from build123d import *

# Parameters (mm, degrees)
SKETCH_1_R          = 140
EXTRUDE_1_DEPTH     = 100
SKETCH_2_R          = 105
CUT_EXTRUDE_1_DEPTH = 100
SKETCH_3_R          = 20
EXTRUDE_2_DEPTH     = 100
SKETCH_4_R          = 130
CUT_EXTRUDE_2_DEPTH = 10
CUT_EXTRUDE_START   = -10
SKETCH_5_R          = 130
CUT_EXTRUDE_3_DEPTH = 10
CUT_EXTRUDE_4_DEPTH = 218.485631709
SKETCH_7_W          = 8
SKETCH_7_H          = 10
SKETCH_7_W_2        = 10
SKETCH_7_H_2        = 8
EXTRUDE_3_DEPTH     = 70
EXTRUDE_4_DEPTH     = 70
FILLET_3_R          = 5
CHAMFER_1_SIZE      = 10
CUT_EXTRUDE_6_DEPTH = 235.447678383
FILLET_4_R          = 10


with BuildPart() as part:
    # 草图1 → 凸台-拉伸1 (new body)
    with BuildSketch(Plane.XY):
        Circle(SKETCH_1_R)
    extrude(amount=EXTRUDE_1_DEPTH)

    # 草图2 → 切除-拉伸1 (cut)
    with BuildSketch(Plane.XY.offset(100)):
        Circle(SKETCH_2_R)
    extrude(amount=-CUT_EXTRUDE_1_DEPTH, mode=Mode.SUBTRACT)

    # 草图3 → 凸台-拉伸2 (add, through all)
    with BuildSketch(Plane.XY.offset(100)):
        with Locations((0, 115)):
            Circle(SKETCH_3_R)
        with Locations((57.5, 99.592921435)):
            Circle(SKETCH_3_R)
        with Locations((99.592921435, 57.5)):
            Circle(SKETCH_3_R)
        with Locations((115, 0)):
            Circle(SKETCH_3_R)
        with Locations((99.592921435, -57.5)):
            Circle(SKETCH_3_R)
        with Locations((57.5, -99.592921435)):
            Circle(SKETCH_3_R)
        with Locations((0, -115)):
            Circle(SKETCH_3_R)
        with Locations((-57.5, -99.592921435)):
            Circle(SKETCH_3_R)
        with Locations((-99.592921435, -57.5)):
            Circle(SKETCH_3_R)
        with Locations((-115, 0)):
            Circle(SKETCH_3_R)
        with Locations((-99.592921435, 57.5)):
            Circle(SKETCH_3_R)
        with Locations((-57.5, 99.592921435)):
            Circle(SKETCH_3_R)
    extrude(amount=-EXTRUDE_2_DEPTH)

    # 草图4 → 切除-拉伸2 (cut)
    with BuildSketch(Plane.XY.offset(100)):
        Circle(SKETCH_4_R)
    extrude(amount=-CUT_EXTRUDE_2_DEPTH, mode=Mode.SUBTRACT)

    # 草图5 → 切除-拉伸3 (cut)
    with BuildSketch(Plane(origin=(0, 0, 0), x_dir=(-1, 0, 0), z_dir=(0, 0, -1)).offset(CUT_EXTRUDE_START)):
        with Locations(Location((0, 0, 0), (0, 0, 180))):
            Circle(SKETCH_5_R)
    extrude(amount=CUT_EXTRUDE_3_DEPTH, mode=Mode.SUBTRACT)

    # 草图6 → 切除-拉伸4 (cut, through all)
    with BuildSketch(Plane.XY.offset(90)):
        Polygon((55.132863896, 95.492921435), (59.867136104, 95.492921435), (62.234272207, 99.592921435), (59.867136104, 103.692921435), (55.132863896, 103.692921435), (52.765727793, 99.592921435), align=None)
        Polygon((0, 110.265727793), (4.1, 112.632863896), (4.1, 117.367136104), (0, 119.734272207), (-4.1, 117.367136104), (-4.1, 112.632863896), align=None)
        Polygon((95.492921435, 55.132863896), (99.592921435, 52.765727793), (103.692921435, 55.132863896), (103.692921435, 59.867136104), (99.592921435, 62.234272207), (95.492921435, 59.867136104), align=None)
        Polygon((110.265727793, 0), (112.632863896, -4.1), (117.367136104, -4.1), (119.734272207, 0), (117.367136104, 4.1), (112.632863896, 4.1), align=None)
        Polygon((95.492921435, -55.132863896), (95.492921435, -59.867136104), (99.592921435, -62.234272207), (103.692921435, -59.867136104), (103.692921435, -55.132863896), (99.592921435, -52.765727793), align=None)
        Polygon((55.132863896, -95.492921435), (52.765727793, -99.592921435), (55.132863896, -103.692921435), (59.867136104, -103.692921435), (62.234272207, -99.592921435), (59.867136104, -95.492921435), align=None)
        Polygon((0, -110.265727793), (-4.1, -112.632863896), (-4.1, -117.367136104), (0, -119.734272207), (4.1, -117.367136104), (4.1, -112.632863896), align=None)
        Polygon((-55.132863896, -95.492921435), (-59.867136104, -95.492921435), (-62.234272207, -99.592921435), (-59.867136104, -103.692921435), (-55.132863896, -103.692921435), (-52.765727793, -99.592921435), align=None)
        Polygon((-95.492921435, -55.132863896), (-99.592921435, -52.765727793), (-103.692921435, -55.132863896), (-103.692921435, -59.867136104), (-99.592921435, -62.234272207), (-95.492921435, -59.867136104), align=None)
        Polygon((-110.265727793, 0), (-112.632863896, 4.1), (-117.367136104, 4.1), (-119.734272207, 0), (-117.367136104, -4.1), (-112.632863896, -4.1), align=None)
        Polygon((-95.492921435, 55.132863896), (-95.492921435, 59.867136104), (-99.592921435, 62.234272207), (-103.692921435, 59.867136104), (-103.692921435, 55.132863896), (-99.592921435, 52.765727793), align=None)
        Polygon((-55.132863896, 95.492921435), (-52.765727793, 99.592921435), (-55.132863896, 103.692921435), (-59.867136104, 103.692921435), (-62.234272207, 99.592921435), (-59.867136104, 95.492921435), align=None)
    extrude(amount=-CUT_EXTRUDE_4_DEPTH, mode=Mode.SUBTRACT)

    # 草图7 → 凸台-拉伸3 (add)
    with BuildSketch(Plane.XY.offset(100)):
        Polygon((66.507321123, 123.19405926), (73.435524353, 119.19405926), (78.435524353, 127.854313298), (71.507321123, 131.854313298), align=None)
        with Locations((0, 144.942845476)):
            Rectangle(SKETCH_7_W, SKETCH_7_H)
        Polygon((119.19405926, 73.435524353), (123.19405926, 66.507321123), (131.854313298, 71.507321123), (127.854313298, 78.435524353), align=None)
        with Locations((144.942845476, 0)):
            Rectangle(SKETCH_7_W_2, SKETCH_7_H_2)
        Polygon((123.19405926, -66.507321123), (119.19405926, -73.435524353), (127.854313298, -78.435524353), (131.854313298, -71.507321123), align=None)
        Polygon((73.435524353, -119.19405926), (66.507321123, -123.19405926), (71.507321123, -131.854313298), (78.435524353, -127.854313298), align=None)
        with Locations((0, -144.942845476)):
            Rectangle(SKETCH_7_W, SKETCH_7_H)
        Polygon((-66.507321123, -123.19405926), (-73.435524353, -119.19405926), (-78.435524353, -127.854313298), (-71.507321123, -131.854313298), align=None)
        Polygon((-119.19405926, -73.435524353), (-123.19405926, -66.507321123), (-131.854313298, -71.507321123), (-127.854313298, -78.435524353), align=None)
        with Locations((-144.942845476, 0)):
            Rectangle(SKETCH_7_W_2, SKETCH_7_H_2)
        Polygon((-123.19405926, 66.507321123), (-119.19405926, 73.435524353), (-127.854313298, 78.435524353), (-131.854313298, 71.507321123), align=None)
        Polygon((-73.435524353, 119.19405926), (-66.507321123, 123.19405926), (-71.507321123, 131.854313298), (-78.435524353, 127.854313298), align=None)
    extrude(amount=-EXTRUDE_3_DEPTH)

    # 草图9 → 凸台-拉伸4 (add)
    with BuildSketch(Plane(origin=(0, 0, 0), x_dir=(-1, 0, 0), z_dir=(0, 0, -1))):
        Polygon((34.944360781, 145.868943093), (32.35617033, 136.20968483), (40.08357694, 134.13913247), (42.671767391, 143.798390732), align=None)
        Polygon((101.78296214, 96.12610789), (108.854029951, 103.197175702), (103.197175702, 108.854029951), (96.12610789, 101.78296214), align=None)
        Polygon((136.20968483, 32.35617033), (145.868943093, 34.944360781), (143.798390732, 42.671767391), (134.13913247, 40.08357694), align=None)
        Polygon((134.13913247, -40.08357694), (143.798390732, -42.671767391), (145.868943093, -34.944360781), (136.20968483, -32.35617033), align=None)
        Polygon((96.12610789, -101.78296214), (103.197175702, -108.854029951), (108.854029951, -103.197175702), (101.78296214, -96.12610789), align=None)
        Polygon((32.35617033, -136.20968483), (34.944360781, -145.868943093), (42.671767391, -143.798390732), (40.08357694, -134.13913247), align=None)
        Polygon((-40.08357694, -134.13913247), (-42.671767391, -143.798390732), (-34.944360781, -145.868943093), (-32.35617033, -136.20968483), align=None)
        Polygon((-101.78296214, -96.12610789), (-108.854029951, -103.197175702), (-103.197175702, -108.854029951), (-96.12610789, -101.78296214), align=None)
        Polygon((-136.20968483, -32.35617033), (-145.868943093, -34.944360781), (-143.798390732, -42.671767391), (-134.13913247, -40.08357694), align=None)
        Polygon((-134.13913247, 40.08357694), (-143.798390732, 42.671767391), (-145.868943093, 34.944360781), (-136.20968483, 32.35617033), align=None)
        Polygon((-96.12610789, 101.78296214), (-103.197175702, 108.854029951), (-108.854029951, 103.197175702), (-101.78296214, 96.12610789), align=None)
        Polygon((-32.35617033, 136.20968483), (-34.944360781, 145.868943093), (-42.671767391, 143.798390732), (-40.08357694, 134.13913247), align=None)
    extrude(amount=-EXTRUDE_4_DEPTH)

    # 圆角3
    fillet_3_edges = [part.edges().sort_by_distance(p)[0] for p in [
        (70, 121.24355653, 30),
        (-70, 121.24355653, 30),
        (-121.24355653, 70, 30),
        (-140, 0, 30),
        (0, 140, 30),
        (121.24355653, 70, 30),
        (139.98571064, 2.000204155, 30),
        (121.24355653, -70, 30),
        (70, -121.24355653, 30),
        (0, -140, 30),
        (-70, -121.24355653, 30),
        (-121.24355653, -70, 30),
        (-119.19405926, -73.435524353, 65),
        (-123.19405926, -66.507321123, 65),
        (-66.507321123, -123.19405926, 65),
        (-73.435524353, -119.19405926, 65),
        (4, -139.942845476, 65),
        (-4, -139.942845476, 65),
        (73.435524353, -119.19405926, 65),
        (66.507321123, -123.19405926, 65),
        (123.19405926, -66.507321123, 65),
        (119.19405926, -73.435524353, 65),
        (139.942845476, 4, 65),
        (139.942845476, -4, 65),
        (119.19405926, 73.435524353, 65),
        (123.19405926, 66.507321123, 65),
        (-4, 139.942845476, 65),
        (4, 139.942845476, 65),
        (-139.942845476, -4, 65),
        (-139.942845476, 4, 65),
        (-123.19405926, 66.507321123, 65),
        (-119.19405926, 73.435524353, 65),
        (-73.435524353, 119.19405926, 65),
        (-66.507321123, 123.19405926, 65),
        (66.507321123, 123.19405926, 65),
        (73.435524353, 119.19405926, 65),
        (-36.234666314, 135.22961568, 70),
        (36.234666314, 135.22961568, 70),
        (98.994949366, 98.994949366, 70),
        (135.22961568, 36.234666314, 70),
        (135.22961568, -36.234666314, 70),
        (98.994949366, -98.994949366, 70),
        (36.234666314, -135.22961568, 70),
        (-36.234666314, -135.22961568, 70),
        (-98.994949366, -98.994949366, 70),
        (-135.22961568, -36.234666314, 70),
        (-135.22961568, 36.234666314, 70),
        (-98.994949366, 98.994949366, 70),
        (-96.12610789, 101.78296214, 35),
        (-101.78296214, 96.12610789, 35),
        (-134.13913247, 40.08357694, 35),
        (-136.20968483, 32.35617033, 35),
        (-136.20968483, -32.35617033, 35),
        (-134.13913247, -40.08357694, 35),
        (-101.78296214, -96.12610789, 35),
        (-96.12610789, -101.78296214, 35),
        (-40.08357694, -134.13913247, 35),
        (-32.35617033, -136.20968483, 35),
        (32.35617033, -136.20968483, 35),
        (40.08357694, -134.13913247, 35),
        (96.12610789, -101.78296214, 35),
        (101.78296214, -96.12610789, 35),
        (134.13913247, -40.08357694, 35),
        (136.20968483, -32.35617033, 35),
        (136.20968483, 32.35617033, 35),
        (134.13913247, 40.08357694, 35),
        (101.78296214, 96.12610789, 35),
        (96.12610789, 101.78296214, 35),
        (40.08357694, 134.13913247, 35),
        (32.35617033, 136.20968483, 35),
        (-40.08357694, 134.13913247, 35),
        (-32.35617033, 136.20968483, 35),
    ]]
    fillet(fillet_3_edges, radius=FILLET_3_R)

    # 倒角1
    chamfer_1_edges = [part.edges().sort_by_distance(p)[0] for p in [
        (74.971422738, 129.854313298, 100),
        (106.025602827, 106.025602827, 0),
        (129.854313298, 74.971422738, 100),
        (144.833666913, 38.808064086, 0),
        (149.942845476, 0, 100),
        (144.833666913, -38.808064086, 0),
        (129.854313298, -74.971422738, 100),
        (106.025602827, -106.025602827, 0),
        (74.971422738, -129.854313298, 100),
        (38.808064086, -144.833666913, 0),
        (0, -149.942845476, 100),
        (-38.808064086, -144.833666913, 0),
        (-74.971422738, -129.854313298, 100),
        (-106.025602827, -106.025602827, 0),
        (-129.854313298, -74.971422738, 100),
        (-144.833666913, -38.808064086, 0),
        (-149.942845476, 0, 100),
        (-129.854313298, 74.971422738, 100),
        (-74.971422738, 129.854313298, 100),
        (0, 149.942845476, 100),
        (-144.833666913, 38.808064086, 0),
        (-106.025602827, 106.025602827, 0),
        (-38.808064086, 144.833666913, 0),
        (38.808064086, 144.833666913, 0),
    ]]
    chamfer(chamfer_1_edges, length=CHAMFER_1_SIZE)

    # 草图10 → 切除-拉伸6 (cut, through all)
    with BuildSketch(Plane(origin=(0, 0, 0), x_dir=(-1, 0, 0), z_dir=(0, 0, -1))):
        with BuildLine():
            Line((0, 0), (25.926748518, 162.950310559))
            ThreePointArc((25.926748518, 162.950310559), (59.021932425, -154.082482758), (-128.15573424, 103.928378134))
            Line((-128.15573424, 103.928378134), (0, 0))
        make_face()
    extrude(amount=-CUT_EXTRUDE_6_DEPTH, mode=Mode.SUBTRACT)

    # 圆角4
    fillet_4_edges = [part.edges().sort_by_distance(p)[0] for p in [
        (81.553649062, 66.136240631, 50),
        (-16.498839966, 103.695652174, 50),
    ]]
    fillet(fillet_4_edges, radius=FILLET_4_R)


solid = part.part
Can you work these out from the model? Positions are in its coordinate system, mm. A direction names the side the tool comes from. Coordinates: 2 decimals unless noted, no trailing zeros. Loops run counter-clockwise (first coordinate to the right, second up) from the corner with the lowest first, then second, coordinate; pieces in that order, holes last. Notation, with made-up numbers: (16, 40.5) - (37, 40.5) arc R25 cw to (37, 55.5) - close; hole circle Ø9 at (55.25, 49.5). An arc over 180 degrees is marked (long way). Answer as a JSON object with one key per item and string values. Group by question number.
Item 1: If we section it at B-B (x = 10.5): List the corners of the cut face in (y, z) for me, plus the area to 3 significant figures.
Item 2: On a 3-axis mill with a long thin cutter (end or side, diameter ignored), from which of +Z, -Z, +X, -X, +Y, -Y can I reach the whole of each face in a straight line? I mean faces 1 (the face through (-4, 147, 63)), 2 (the face through (104, 104, 70)), 3 (the face through (71.01, 77.347, 50.56)), 4 (the face through (-4.1, 115, 51)). Say none if no direction works.
Item 3: If we section it at A-A (z = 11.5): State how many separate pieces and enclosed holes the cut face has, plus the area to 3 significant figures.
Item 4: For pin 1 (2 mm diameter, centred on x = 39.5, y = 143, fed in from +Z); pin 2 (12 mm diameter, centred on y = 117.5, z = 12.5, fed in from +X); pin 3 (4 mm diameter, centred on x = 57.5, z = 44, fed in from -Y); pin 4 (1.5 mm diameter, centred on x = -1.5, y = 140.5, fed in from +Z), each with a flat end and sliding along its axis, tell me the tip position at first contact or that it passes through.
Item 5: If we mould it in two halves opening along Y, with no side actions, what happens to faces 5 (the face through (65.96, 125.03, 61.98)), 6 (the face through (61.07, 101.61, 50.56)), 7 (the face through (-2.02, 118.57, 50.56)), 8 (the face through (1.641, 95.067, 50.56))? For each: released by +Y, released by -Y, zero draft, split by the parting line, or undercut.
Item 6: If I drill on L1, parallel to X at y = 97, z = 13.5; L2, parallel to Z at x = 67, y = 106; L3, parallel to X at y = 115.5, z = 68, over which ranges is the centre line in solid material (lowest first)? Write a range as from..to.
Item 7: If we section it at C-C (y = 77): List the corners of the cut face in (x, z) for me, plus the area to 3 significant figures.
Returned:
{
 "1": {"outline": "(97.98, 10) - (129.58, 10) - (129.58, 0) - (139.61, 0) - (139.61, 100) - (129.58, 100) - (129.58, 90) - (97.98, 90) - close", "area": "3,530 mm²"},
 "2": {"face 1": "+Z, -Z, -X, +Y", "face 2": "+Z, +X, +Y", "face 3": "+Z, -Z, -Y", "face 4": "+Z, -Z"},
 "3": {"separate pieces": "1", "enclosed holes": "2", "area": "4,990 mm²"},
 "4": {"pin 1": "stops at z = 70", "pin 2": "stops at x = 84.66", "pin 3": "stops at y = 79.59", "pin 4": "stops at z = 100"},
 "5": {"face 5": "released by +Y", "face 6": "undercut", "face 7": "undercut", "face 8": "released by -Y"},
 "6": {"L1": "x = -8.72..8.72, 37.67..54.26, 60.74..103.8", "L2": "z = 10..90", "L3": "x = -18.38..-4.1, 4.1..79.12"},
 "7": {"outline": "(71.39, 10) - (94.95, 10) - (94.95, 90) - (71.39, 90) - close", "area": "1,890 mm²"}
}
